```python
from build123d import *

# Parameters (mm, degrees)
BOSS_EXTRUDE1_DEPTH = 150
SKETCH2_W           = 1.5
SKETCH2_H           = 9
BOSS_EXTRUDE2_DEPTH = 2.8
SKETCH4_W           = 16
SKETCH4_H           = 3
SKETCH4_W_2         = 11
SKETCH4_H_2         = 19.5
CUT_EXTRUDE2_DEPTH  = 22
CHAMFER1_SIZE       = 2


with BuildPart() as part:
    # Sketch1 → Boss-Extrude1 (new body)
    with BuildSketch(Plane(origin=(0, 0, 0), x_dir=(0, 0, -1), z_dir=(1, 0, 0))):
        Polygon((0, 0), (-16.5, 0), (-16.5, 1.5), (-2, 1.5), (-2, 4), (-2, 7.35), (1, 7.35), (1, 5.85), (0, 5.85), (0, 4), (3, 4), (3, 0), align=None)
    extrude(amount=BOSS_EXTRUDE1_DEPTH)

    # Sketch2 → Boss-Extrude2 (add)
    with BuildSketch(Plane(origin=(0, 1.5, 0), x_dir=(1, 0, 0), z_dir=(0, 1, 0))):
        with Locations((33.75, -12)):
            Rectangle(SKETCH2_W, SKETCH2_H)
        with Locations((46.25, -12)):
            Rectangle(SKETCH2_W, SKETCH2_H)
        with Locations((103.75, -12)):
            Rectangle(SKETCH2_W, SKETCH2_H)
        with Locations((116.25, -12)):
            Rectangle(SKETCH2_W, SKETCH2_H)
    extrude(amount=BOSS_EXTRUDE2_DEPTH)

    # Sketch4 → Cut-Extrude2 (cut)
    with BuildSketch(Plane(origin=(0, 7.35, 0), x_dir=(1, 0, 0), z_dir=(0, 1, 0))):
        with Locations((25, 1.5)):
            Rectangle(SKETCH4_W, SKETCH4_H)
        with Locations((144.5, -6.75)):
            Rectangle(SKETCH4_W_2, SKETCH4_H_2)
    extrude(amount=-CUT_EXTRUDE2_DEPTH, mode=Mode.SUBTRACT)

    # Chamfer1
    chamfer1_edges = [part.edges().sort_by_distance(p)[0] for p in [
        (33.75, 4.3, 16.5),
        (46.25, 4.3, 16.5),
        (103.75, 4.3, 16.5),
        (116.25, 4.3, 16.5),
    ]]
    chamfer(chamfer1_edges, length=CHAMFER1_SIZE)


solid = part.part
```
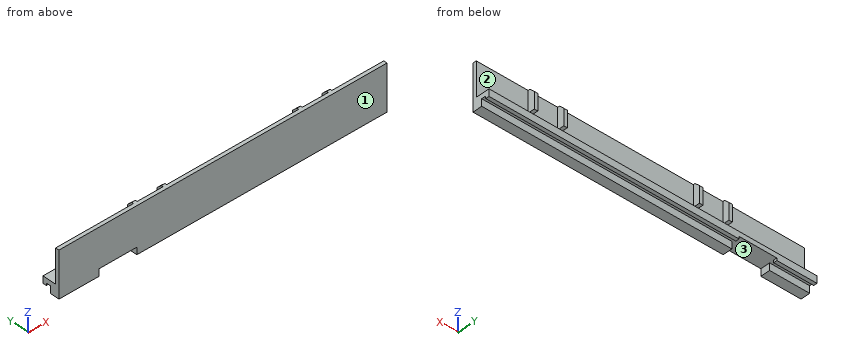
Input: part model. Units: mm. Frame: model coordinates. Face numbers are marked on the shaded views. Give positions to 0.01 mm unless a question says otherwise; leave off trailing zeros. Loops run counter-clockwise (first coordinate to the right, second up) from the corner with the lowest first, then second, coordinate; pieces in that order, holes last. Notation, with made-up numbers: M 14.5,76.25 L 54.5,76.25 A18 cw 54.5,97.25 Z; hole C -18.75,19.25 d10. An arc over 180 degrees is marked long. Answer as CSV lines item,"result". Start each with the question number.
1. Section A-A on x = 58.5. Return loops of the section in (y, z).
2. Pull-direction query (X, two-part tool) for the marked faces 1, 2 and 3; classes: released by +X, released by -X, zero draft, split by the parting line, or undercut.
3. Section B-B on z = 5.25. Return loops of the section in (x, y), plus the area to 4 significant figures.
4. Line query: L1, parallel to X at y = 1.75, z = 11.5; L2, parallel to X at y = 0.5, z = -1.5; L3, parallel to Z at x = 24, y = 1.75. Output: solid intervals per line, ascending.
5. Pin query (flat end, axial travel): P1, Ø1.2, axis at x = 112, y = 6.5, coming from the -Z side; P2, Ø1.8, axis at x = 63.5, y = 5, coming from the +Z side; P3, Ø2, axis at y = 3.5, z = 10.5, coming from the +X side. Return the tip coordinate at first contact, or that it passes through.
Computed values:
1,outline,"M 0,-3 L 4,-3 L 4,0 L 5.85,0 L 5.85,-1 L 7.35,-1 L 7.35,2 L 1.5,2 L 1.5,16.5 L 0,16.5 Z"
2,face 1,"zero draft"
2,face 2,"undercut"
2,face 3,"undercut"
3,outline,"M 0,0 L 139,0 L 139,1.5 L 0,1.5 Z"
3,area,"208.5 mm²"
4,L1,"x = 33 to 34.5, 45.5 to 47, 103 to 104.5, 115.5 to 117"
4,L2,"x = 0 to 17, 33 to 139"
4,L3,"z = 0 to 2"
5,P1,"stops at z = -1"
5,P2,"stops at z = 2"
5,P3,"stops at x = 117"
